Verification items for the finished model (mm, model axes). A direction names the side the tool comes from. Round coordinates to 2 decimals unless told otherwise and drop trailing zeros. Write each loop counter-clockwise with the first axis right and the second up, starting at its lowest first coordinate (ties: lowest second). Pieces come first, ordered by that corner, then holes. Notation, with made-up numbers: M 62,84 L 117,84 A26 ccw 117,118 Z; hole C 73,27.5 d9. An arc over 180 degrees is marked long. One line per question, with ' | ' between items.
from build123d import *

# Parameters (mm, degrees)
SKETCH_R        = 20.5
PAD_DEPTH       = 17
SKETCH001_R     = 19.75
POCKET_DEPTH    = 15
SKETCH002_W     = 21
SKETCH002_H     = 2
POCKET001_DEPTH = 5
SKETCH003_R     = 5.8
PAD001_DEPTH    = 10
SKETCH004_R     = 4.75
POCKET002_DEPTH = 13
SKETCH005_W     = 22.5
SKETCH005_H     = 1.5
SKETCH005_W_2   = 1.5
SKETCH005_H_2   = 3.5
PAD002_DEPTH    = 3


with BuildPart() as part:
    # Sketch → Pad (new body)
    with BuildSketch(Plane.XY):
        Circle(SKETCH_R)
    extrude(amount=PAD_DEPTH)

    # Sketch001 (on Face3 of Pad) → Pocket (cut)
    with BuildSketch(Plane.XY.offset(17)):
        Circle(SKETCH001_R)
    extrude(amount=-POCKET_DEPTH, mode=Mode.SUBTRACT)

    # Sketch002 (on Face5 of Pocket) → Pocket001 (cut)
    with BuildSketch(Plane.XY.offset(2)):
        Rectangle(SKETCH002_W, SKETCH002_H)
    extrude(amount=-POCKET001_DEPTH, mode=Mode.SUBTRACT)

    # Sketch003 (on Face9 of Pocket001) → Pad001 (join)
    with BuildSketch(Plane.XY.offset(2)):
        with Locations((0, 12)):
            Circle(SKETCH003_R)
    extrude(amount=PAD001_DEPTH)

    # Sketch004 (on Face11 of Pad001) → Pocket002 (cut)
    with BuildSketch(Plane.XY.offset(12)):
        with Locations((0, 12)):
            Circle(SKETCH004_R)
    extrude(amount=-POCKET002_DEPTH, mode=Mode.SUBTRACT)

    # Sketch005 (on Face10 of Pocket002) → Pad002 (join)
    with BuildSketch(Plane.XY.offset(2)):
        with Locations((-0.75, 1.75)):
            Rectangle(SKETCH005_W, SKETCH005_H)
        with Locations((11.25, 0.75)):
            Rectangle(SKETCH005_W_2, SKETCH005_H_2)
        with Locations((0.75, -1.75)):
            Rectangle(SKETCH005_W, SKETCH005_H)
        with Locations((-11.25, -0.75)):
            Rectangle(SKETCH005_W_2, SKETCH005_H_2)
    extrude(amount=PAD002_DEPTH)


solid = part.part
1. Section check D-D, the plane z = 11. Record the cut outline in (x, y), then the cut area to 3 significant figures.
Results:
outline: C 0,0 d41; C 0,12 d11.6; hole C 0,0 d39.5; hole C 0,12 d9.5 | area: 130 mm2
2. Tool access check on faces 1 (the face through (12, 0, 3)), 2 (the face through (0, 1, 2)), 3 (the face through (0, -4, 0)). Record the directions out of +Z, -Z, +X, -X, +Y, -Y that give a thin tool (end or side, any length) a straight path to the whole face; none if there is none.
Results:
face 1: +Z | face 2: +Z, -Z | face 3: -Z, +X, -X, +Y, -Y
3. Mould release check, pull along Y, two halves, no side actions. Record for faces 4 (the face through (0, 2.5, 3)), 5 (the face through (-4.444, -20.013, 8.381)), 6 (the face through (-11, 17, 17)): pulls with the +Y half, pulls with the -Y half, needs draft (parallel to the pull), parting line crosses it, or undercut.
Results:
face 4: undercut | face 5: parting line crosses it | face 6: needs draft
4. Thickness scan on line 1 (Y direction, x = 0, z = 7.75); line 2 (X direction, y = 10.5, z = 10); line 3 (Y direction, x = -1.5, z = 4). Record the ranges inside material, lowest first.
Results:
line 1: y = -20.5 to -19.75, 6.2 to 7.25, 16.75 to 17.8, 19.75 to 20.5 | line 2: x = -17.61 to -16.73, -5.6 to -4.51, 4.51 to 5.6, 16.73 to 17.61 | line 3: y = -20.45 to -19.69, -2.5 to -1, 1 to 2.5, 6.4 to 7.49, 16.51 to 17.6, 19.69 to 20.45
5. Section check B-B, the plane y = 0. Record the cut outline in (x, z), then the cut area to 3 significant figures.
Results:
outline: M -20.5,0 L -10.5,0 L -10.5,5 L -12,5 L -12,2 L -19.75,2 L -19.75,17 L -20.5,17 Z; M 10.5,0 L 20.5,0 L 20.5,17 L 19.75,17 L 19.75,2 L 12,2 L 12,5 L 10.5,5 Z | area: 71.5 mm2
6. Section check C-C, the plane x = 0. Record the cut outline in (y, z).
Results:
outline: M -20.5,0 L -1,0 L -1,5 L -2.5,5 L -2.5,2 L -19.75,2 L -19.75,17 L -20.5,17 Z; M 1,0 L 7.25,0 L 7.25,12 L 6.2,12 L 6.2,2 L 2.5,2 L 2.5,5 L 1,5 Z; M 16.75,0 L 20.5,0 L 20.5,17 L 19.75,17 L 19.75,2 L 17.8,2 L 17.8,12 L 16.75,12 Z
7. Section check A-A, the plane z = 2.5. Record the cut outline in (x, y), then the cut area to 3 significant figures.
Results:
outline: C 0,0 d41; M -12,-2.5 L 12,-2.5 L 12,2.5 L -12,2.5 Z; C 0,12 d11.6; hole C 0,0 d39.5; hole M -10.5,-1 L 10.5,-1 L 10.5,1 L -10.5,1 Z; hole C 0,12 d9.5 | area: 208 mm2
8. Go/stop test with flat-tipped pins: P1, Ø2.5, axis at x = 5, z = 1.5, coming from the -Y side; P2, Ø5, axis at y = -14.5, z = 12, coming from the +X side; P3, Ø6, axis at x = 1, z = 2, coming from the +Y side; P4, Ø1, axis at x = -13, y = 15.5, coming from the -Z side. Record where each tip stops, or that it passes through.
Results:
P1: stops at y = -20.15 | P2: stops at x = 16.62 | P3: stops at y = 20.5 | P4: stops at z = 0
